Verification items for the finished model (mm, model axes). Coordinates: 2 decimals unless noted, no trailing zeros. Order: outer loops, then holes, each group sorted by start corner. A loop starts at its lowest first (then second) coordinate and runs counter-clockwise, first axis right, second up.
Q1. Cross-section at A-A, the plane z = 37. Record the boundary of the cut face in (x, y), and give its area (3 significant figures).
Q2. Cross-section at B-B, the plane x = -37. Record the boundary of the cut face in (y, z), and give its area (3 significant figures).
Q3. Cross-section at C-C, the plane y = -1.25. Count the separate pieces of the cut face and the enclosed holes in it, and give its area (3 significant figures).
Q4. Thickness scan on line 1 (Z direction, x = 4.5, y = -1.75); line 2 (Z direction, x = -28.5, y = -1.1); line 3 (Z direction, x = -21, y = -0.75). Record the ranges inside material, lowest first.
Q5. Cross-section at D-D, the plane x = -21. Record the boundary of the cut face in (y, z).
Q6. Depth check by flat-ended pin: P1, Ø5.5, axis at x = 0, z = -37, coming from the +Y side. Enter the tip coordinate at first touch or a pass-through.
Q7. Draft check along Z on faces 1 (the flat face through (19, -3, -18)), 2 (the cylindrical face through (-34.9, -2.44, 0.09)). Enter one of: pulls with the +Z half, pulls with the -Z half, needs draft (parallel to the pull), parting line crosses it, or undercut.
Autodesk Inventor part; units mm, degrees
ref_plane "YZ Plane" through (0, 0, 0) normal (1, 0, 0) x (0, 1, 0)
ref_plane "XZ Plane" through (0, 0, 0) normal (0, 1, 0) x (-1, 0, 0)
ref_plane "XY Plane" through (0, 0, 0) normal (0, 0, 1) x (1, 0, 0)
sketch "Sketch1" plane through (0, 0, 0) normal (0, 1, 0) x (-1, 0, 0)
  circle A0 centre (0, 0) radius 42
  circle A1 centre (0, 0) radius 19.5
  circle A2 centre (0, -37) radius 2.1
  circle A3 centre (26.163, -26.163) radius 2.1
  circle A4 centre (37, 0) radius 2.1
  circle A5 centre (26.163, 26.163) radius 2.1
  circle A6 centre (0, 37) radius 2.1
  circle A7 centre (-26.163, 26.163) radius 2.1
  circle A8 centre (-37, 0) radius 2.1
  circle A9 centre (-26.163, -26.163) radius 2.1
  dimension "d0" = 84
  dimension "d1" = 39
  dimension "d2" = 4.2
  dimension "d3" = 37
  dimension "d6" = 360
extrude "Extrusion1" add sketch "Sketch1" against normal blind 3
sketch "Sketch2" plane through (0, -3, 0) normal (0, -1, 0) x (1, 0, 0)
  circle A0 centre (0, 0) radius 24
  dimension "d10" = 48
extrude "Extrusion2" cut sketch "Sketch2" against normal blind 1
hole "Hole1" at (37, 0, 0) at (26.163, 0, 26.163) at (0, 0, 37) at (-26.163, 0, 26.163) at (-37, 0, 0) at (-26.163, 0, -26.163) at (0, 0, -37) at (26.163, 0, -26.163) direction (0, -1, 0) diameter 4.2 end through all countersink diameter 8 countersink angle 90
sketch "Sketch3" plane through (0, 0, 0) normal (0, 1, 0) x (1, 0, 0)
  circle A0 centre (-4.8621, -27.5746) radius 2.1
  circle A1 centre (4.8621, -27.5746) radius 2.1
  circle A2 centre (14, -24.2487) radius 2.1
  circle A3 centre (21.4492, -17.9981) radius 2.1
  circle A4 centre (26.3114, -9.5766) radius 2.1
  circle A5 centre (28, 0) radius 2.1
  circle A6 centre (26.3114, 9.5766) radius 2.1
  circle A7 centre (21.4492, 17.9981) radius 2.1
  circle A8 centre (14, 24.2487) radius 2.1
  circle A9 centre (4.8621, 27.5746) radius 2.1
  circle A10 centre (-4.8621, 27.5746) radius 2.1
  circle A11 centre (-14, 24.2487) radius 2.1
  circle A12 centre (-21.4492, 17.9981) radius 2.1
  circle A13 centre (-26.3114, 9.5766) radius 2.1
  circle A14 centre (-28, 0) radius 2.1
  circle A15 centre (-26.3114, -9.5766) radius 2.1
  circle A16 centre (-21.4492, -17.9981) radius 2.1
  circle A17 centre (-14, -24.2487) radius 2.1
  line L0 (0, 0) -> (-4.8621, -27.5746) construction
  line L1 (0, 0) -> (0, -11.0753) construction
  dimension "d20" = 4.2
  dimension "d21" = 28
  dimension "d24" = 360
  dimension "d64" = 10
extrude "Extrusion3" cut sketch "Sketch3" against normal through all
thread "Thread1"
thread "Thread2"
thread "Thread3"
thread "Thread4"
thread "Thread5"
thread "Thread6"
thread "Thread7"
thread "Thread8"
thread "Thread9"
thread "Thread10"
thread "Thread11"
thread "Thread12"
thread "Thread13"
thread "Thread14"
thread "Thread15"
thread "Thread16"
thread "Thread17"
thread "Thread18"
properties part number "HousingLid"
Check values:
1. outline: (-19.87, -3) - (-2.1, -3) - (-2.1, -1.9) - (-4, 0) - (-19.87, 0) - close; (2.1, -3) - (19.87, -3) - (19.87, 0) - (4, 0) - (2.1, -1.9) - close
1. area: 103 mm2
2. outline: (-3, -19.87) - (0, -19.87) - (0, -4) - (-1.9, -2.1) - (-3, -2.1) - close; (-3, 2.1) - (-1.9, 2.1) - (0, 4) - (0, 19.87) - (-3, 19.87) - close
2. area: 103 mm2
3. separate pieces: 1
3. enclosed holes: 27
3. area: 3,910 mm2
4. line 1: z = -41.76 to -29.64, -25.51 to -18.97, 18.97 to 25.51, 29.64 to 41.76
4. line 2: z = -30.85 to -27.88, -24.45 to -2.04, 2.04 to 24.45, 27.88 to 30.85
4. line 3: z = -36.37 to -20.05, -15.95 to 15.95, 20.05 to 36.37
5. outline: (-3, -36.37) - (0, -36.37) - (0, -20.05) - (-3, -20.05) - close; (-3, -15.95) - (0, -15.95) - (0, 15.95) - (-3, 15.95) - (-3, 11.62) - (-2, 11.62) - (-2, -11.62) - (-3, -11.62) - close; (-3, 20.05) - (0, 20.05) - (0, 36.37) - (-3, 36.37) - close
6. P1: stops at y = -1.25
7. face 1: needs draft
7. face 2: undercut
